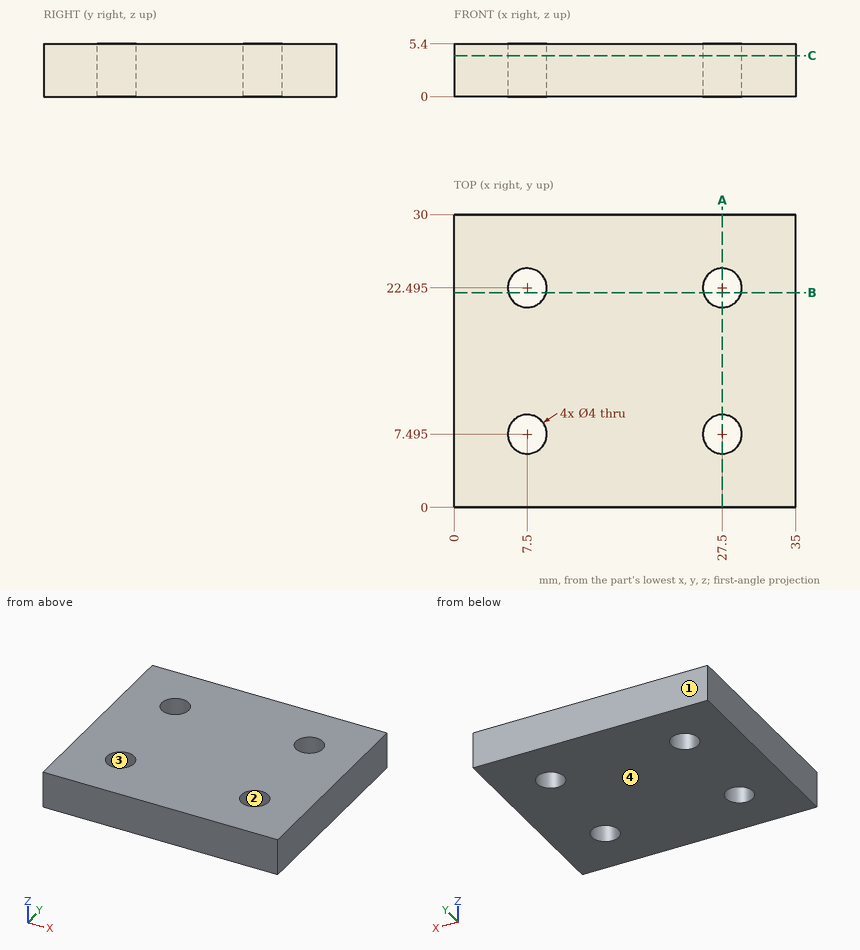
Answer from the drawing. Dimensions are ordinates in mm from the lowest x, y and z of the part. Coordinates: 2 decimals unless noted, no trailing zeros. Order: outer loops, then holes, each group sorted by start corner. A loop starts at its lowest first (then second) coordinate and runs counter-clockwise, first axis right, second up. Notation, with made-up numbers: (71, 31) -> (127, 31) arc R19 cw to (127, 48) -> close; hole circle Ø8 at (-32.75, 71.5). An arc over 180 degrees is marked (long way). Answer as a JSON object with one key per item and string values.
1) A cutting plane is placed at A-A, the plane x = 27.5. Determine the outline of the cut face in (y, z) (3 decimals), plus the area to 3 significant figures.
Model answer:
{"outline": "(0, 0) -> (5.495, 0) -> (5.495, 5.4) -> (0, 5.4) -> close; (9.495, 0) -> (20.495, 0) -> (20.495, 5.4) -> (9.495, 5.4) -> close; (24.495, 0) -> (30, 0) -> (30, 5.4) -> (24.495, 5.4) -> close", "area": "119 mm²"}
2) The mould has two halves that part along Y. Classify the marked faces 1, 2, 3 and 4: released by +Y, released by -Y, zero draft, split by the parting line, or undercut.
Model answer:
{"face 1": "released by +Y", "face 2": "undercut", "face 3": "undercut", "face 4": "zero draft"}
3) A cutting plane is placed at C-C, the plane z = 4.2. Determine the outline of the cut face in (x, y) (3 decimals).
Model answer:
{"outline": "(0, 0) -> (35, 0) -> (35, 30) -> (0, 30) -> close; hole circle Ø4 at (7.5, 7.495); hole circle Ø4 at (7.5, 22.495); hole circle Ø4 at (27.5, 7.495); hole circle Ø4 at (27.5, 22.495)"}
4) Each of these flat-tipped pins is pushed along its axis until it touches: pin 1 (1 mm diameter, centred on y = 5, z = 2, fed in from -X); pin 2 (3 mm diameter, centred on x = 27.5, y = 7.495, fed in from -Z). Where does it stop, or does it pass through?
Model answer:
{"pin 1": "stops at x = 0", "pin 2": "passes through"}
5) A cutting plane is placed at B-B, the plane y = 22. Determine the outline of the cut face in (x, z).
Model answer:
{"outline": "(0, 0) -> (5.56, 0) -> (5.56, 5.4) -> (0, 5.4) -> close; (9.44, 0) -> (25.56, 0) -> (25.56, 5.4) -> (9.44, 5.4) -> close; (29.44, 0) -> (35, 0) -> (35, 5.4) -> (29.44, 5.4) -> close"}
6) Consider line 1 along Y through (x, z) = (7.5, 4.05) (3 decimals); line 2 along X through (y, z) = (23, 2.9); line 3 along X through (y, z) = (24, 5.05). Determine where each line is inside the solid, lowest interval first. Write a range as from..to.
Model answer:
{"line 1": "y = 0..5.495, 9.495..20.495, 24.495..30", "line 2": "x = 0..5.56, 9.44..25.56, 29.44..35", "line 3": "x = 0..6.18, 8.82..26.18, 28.82..35"}
